from build123d import *

# Parameters (mm, degrees)
SKETCH_W        = 50
SKETCH_H        = 39
PAD_DEPTH       = 17.5
SKETCH001_W     = 47
SKETCH001_H     = 36
POCKET_DEPTH    = 16
SKETCH002_W     = 3
SKETCH002_H     = 4
POCKET001_DEPTH = 1.6
SKETCH006_W     = 2
SKETCH006_H     = 12
SKETCH006_H_2   = 14
SKETCH006_H_3   = 18
SKETCH006_H_4   = 16
SKETCH006_H_5   = 13
SKETCH006_H_6   = 15
SKETCH006_H_7   = 17
SKETCH006_H_8   = 11
POCKET002_DEPTH = 1.7
FILLET_R        = 1


with BuildPart() as part:
    # Sketch → Pad (new body)
    with BuildSketch(Plane.XY):
        Rectangle(SKETCH_W, SKETCH_H)
    extrude(amount=PAD_DEPTH)

    # Sketch001 (on Face6 of Pad) → Pocket (cut)
    with BuildSketch(Plane.XY.offset(17.5)):
        Rectangle(SKETCH001_W, SKETCH001_H)
    extrude(amount=-POCKET_DEPTH, mode=Mode.SUBTRACT)

    # Sketch002 (on Face4 of Pocket) → Pocket001 (cut)
    with BuildSketch(Plane(origin=(0, 0, 0), x_dir=(1, 0, 0), z_dir=(0, 0, -1))):
        with Locations((21, 13.5)):
            Rectangle(SKETCH002_W, SKETCH002_H)
        with Locations((21, -13.5)):
            Rectangle(SKETCH002_W, SKETCH002_H)
    extrude(amount=-POCKET001_DEPTH, mode=Mode.SUBTRACT)

    # Sketch006 (on Face4 of Pocket001) → Pocket002 (cut)
    with BuildSketch(Plane(origin=(0, 0, 0), x_dir=(1, 0, 0), z_dir=(0, 0, -1))):
        with Locations((-16, -1)):
            Rectangle(SKETCH006_W, SKETCH006_H)
        with Locations((-12, 0)):
            Rectangle(SKETCH006_W, SKETCH006_H_2)
        with Locations((-8, 2)):
            Rectangle(SKETCH006_W, SKETCH006_H_3)
        with Locations((-4, 1)):
            Rectangle(SKETCH006_W, SKETCH006_H_4)
        with Locations((0, -0.5)):
            Rectangle(SKETCH006_W, SKETCH006_H_5)
        with Locations((4, 0.5)):
            Rectangle(SKETCH006_W, SKETCH006_H_6)
        with Locations((8, 1.5)):
            Rectangle(SKETCH006_W, SKETCH006_H_7)
        with Locations((12, 0.5)):
            Rectangle(SKETCH006_W, SKETCH006_H_6)
        with Locations((16, -1.5)):
            Rectangle(SKETCH006_W, SKETCH006_H_8)
    extrude(amount=-POCKET002_DEPTH, mode=Mode.SUBTRACT)

    # Fillet
    fillet_edges = [part.edges().sort_by_distance(p)[0] for p in [
        (25, -19.5, 8.75),
        (0, -19.5, 0),
        (25, 0, 0),
        (0, 19.5, 0),
        (25, 19.5, 8.75),
        (-25, 0, 0),
        (-25, 19.5, 8.75),
        (-25, -19.5, 8.75),
    ]]
    fillet(fillet_edges, radius=FILLET_R)


solid = part.part
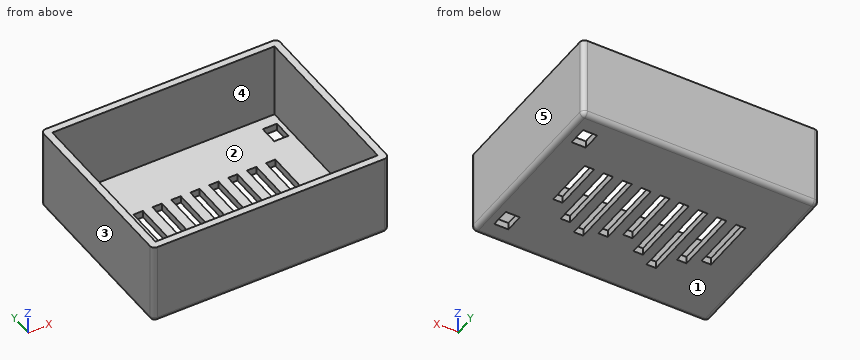
The listing builds one solid part. Answer for the finished solid, in the listing's coordinates (mm). Face numbers are marked on the shaded views. A direction names the side the tool comes from. Round coordinates to 2 decimals unless told otherwise and drop trailing zeros. Order: outer loops, then holes, each group sorted by start corner. A loop starts at its lowest first (then second) coordinate and runs counter-clockwise, first axis right, second up. Notation, with made-up numbers: (33, 16.5) -> (49, 16.5) arc R14 cw to (49, 21.5) -> close; hole circle Ø6 at (19, 48.25). An arc over 180 degrees is marked (long way). Write each question's results on one line, items separated by ' | '. Start each with the question number.
Q1. Find section C-C (y = 12.5). Determine the outline of the cut face in (x, z).
Q2. Find section B-B (z = 15.25). Determine the outline of the cut face in (x, y).
Q3. Find section A-A (x = -4). Determine the outline of the cut face in (y, z), then the cut area to 3 significant figures.
Q4. Straight lines are drawn through the part: probe 1 along Y at (x, z) = (-3.5, 1); probe 2 along Y at (x, z) = (-4, 8); probe 3 along X at (y, z) = (-15, 2). For each, find the intervals that lie inside material, in ascending order. Write a range as from..to.
Q5. Which of the six approach directions +Z, -Z, +X, -X, +Y, -Y give full straight-line access (tool end or side, diameter ignored) to the marked faces 1 and 2?
Q6. The mould has two halves that part along X. Classify the marked faces 3, 4 and 5: pulls with the +X half, pulls with the -X half, needs draft (parallel to the pull), parting line crosses it, or undercut.
Q7. Each of these flat-tipped pins is pushed along its axis until it touches: pin 1 (1.2 mm diameter, centred on y = 1.5, z = 0.5, fed in from -X); pin 2 (2 mm diameter, centred on x = 20, y = -0.5, fed in from +Z); pin 3 (0.8 mm diameter, centred on x = 4, z = 0.5, fed in from -Y) (3 decimals). Where does it stop, or does it pass through?
Q8. Find section D-D (y = 2). Give the number of separate pieces and of enclosed holes in the cut face, then the cut area to 3 significant figures.
Worked answers:
1) outline: (-25, 1) arc R1 ccw to (-24, 0) -> (19.5, 0) -> (19.5, 1.5) -> (-23.5, 1.5) -> (-23.5, 17.5) -> (-25, 17.5) -> close; (22.5, 0) -> (24, 0) arc R1 ccw to (25, 1) -> (25, 17.5) -> (23.5, 17.5) -> (23.5, 1.5) -> (22.5, 1.5) -> close
2) outline: (-25, -18.5) arc R1 ccw to (-24, -19.5) -> (24, -19.5) arc R1 ccw to (25, -18.5) -> (25, 18.5) arc R1 ccw to (24, 19.5) -> (-24, 19.5) arc R1 ccw to (-25, 18.5) -> close; hole (-23.5, -18) -> (23.5, -18) -> (23.5, 18) -> (-23.5, 18) -> close
3) outline: (-19.5, 1) arc R1 ccw to (-18.5, 0) -> (-9, 0) -> (-9, 1.5) -> (-18, 1.5) -> (-18, 17.5) -> (-19.5, 17.5) -> close; (7, 0) -> (18.5, 0) arc R1 ccw to (19.5, 1) -> (19.5, 17.5) -> (18, 17.5) -> (18, 1.5) -> (7, 1.5) -> close | area: 82.1 mm2
4) probe 1: y = -19.5..-9, 7..19.5 | probe 2: y = -19.5..-18, 18..19.5 | probe 3: x = -25..-23.5, 23.5..25
5) face 1: -Z, +X, -X, +Y, -Y | face 2: +Z
6) face 3: pulls with the -X half | face 4: undercut | face 5: pulls with the +X half
7) pin 1: stops at x = -25 | pin 2: stops at z = 1.5 | pin 3: stops at y = -19.495
8) separate pieces: 10 | enclosed holes: 0 | area: 95.6 mm2
